Here's how the part is built. I have some questions about the finished solid (model axes, mm). A direction names the side the tool comes from. Coordinates: 2 decimals unless noted, no trailing zeros. Write each loop counter-clockwise with the first axis right and the second up, starting at its lowest first coordinate (ties: lowest second). Pieces come first, ordered by that corner, then holes. Notation, with made-up numbers: M 75.5,23.5 L 121.5,23.5 A14 ccw 121.5,37.5 Z; hole C 43.25,4.5 d11. An arc over 180 degrees is marked long. Use a Markdown table: item, result.
Solid Edge part; units mm, degrees
sketch "Sketch1" plane through (0, 0, 0) normal (0, -1, 0) x (1, 0, 0)
  line L0 (-16, -36) -> (16, -36)
  line L1 (16, -36) -> (16, 36)
  line L2 (16, 36) -> (-16, 36)
  line L3 (-16, 36) -> (-16, -36)
  line L4 (-20, -40) -> (20, -40)
  line L5 (20, -40) -> (20, 40)
  line L6 (20, 40) -> (-20, 40)
  line L7 (-20, 40) -> (-20, -40)
  dimension "D1" = 20
  dimension "D2" = 20
extrude "Protrusion1" add sketch "Sketch1" along normal mid plane 700
sketch "Sketch2" plane through (-20, 0, 0) normal (-1, 0, 0) x (0, -1, 0)
  line L0 (196, -40) -> (216, -40)
  line L1 (216, -40) -> (216, -35)
  line L2 (216, -35) -> (196, -35)
  line L3 (196, -35) -> (196, -40)
  line L4 (-284, -40) -> (-264, -40)
  line L5 (-264, -40) -> (-264, -35)
  line L6 (-264, -35) -> (-284, -35)
  line L7 (-284, -35) -> (-284, -40)
  dimension "D1" = 264
  dimension "D2" = 264
  dimension "D3" = 216
  dimension "D4" = 196
extrude "Cutout1" cut sketch "Sketch2" against normal through all
sketch "Sketch3" plane through (-20, 0, 0) normal (-1, 0, 0) x (0, -1, 0)
  circle A0 centre (-126, 10) radius 3.5
  circle A1 centre (34, 10) radius 3.5
  dimension "D1" = 126
  dimension "D2" = 126
extrude "Cutout2" cut sketch "Sketch3" against normal through all
sketch "Sketch4" plane through (-20, 0, 0) normal (-1, 0, 0) x (0, -1, 0)
  line L0 (350, 40) -> (313.5, 40)
  line L1 (313.5, 40) -> (313.5, 36)
  line L2 (313.5, 36) -> (346, 36)
  line L3 (346, 36) -> (346, 32)
  line L4 (346, 32) -> (350, 32)
  line L5 (350, 32) -> (350, 40)
  dimension "D1" = 350
  dimension "D2" = 313.5
  dimension "D3" = 346
  dimension "D4" = 346
extrude "Cutout3" cut sketch "Sketch4" against normal through all
mirror "Mirror1" about plane through (0, 0, 0) normal (0, 0, 1) of "Cutout3"
mirror "Mirror2" about plane through (0, 0, 0) normal (0, -1, 0) of "Cutout3", "Mirror1"
sketch "Sketch5" plane through (-20, 0, 0) normal (-1, 0, 0) x (0, 1, 0)
  circle A0 centre (-330, 0) radius 3
  circle A1 centre (-300, -25) radius 3
  circle A2 centre (-300, 25) radius 3
  dimension "D1" = 330
extrude "Cutout4" cut sketch "Sketch5" against normal through all
mirror "Mirror3" about plane through (0, 0, 0) normal (0, -1, 0) of "Cutout4"
sketch "Sketch6" plane through (-20, 0, 0) normal (-1, 0, 0) x (0, -1, 0)
  circle A0 centre (241, -27.5) radius 4
  circle A1 centre (241, -9.5) radius 3.25
  circle A2 centre (215, -27.5) radius 3.25
  circle A3 centre (215, -9.5) radius 4
  circle A4 centre (129, -9.5) radius 4
  circle A5 centre (103, -9.5) radius 3.25
  circle A6 centre (103, -27.5) radius 4
  circle A7 centre (129, -27.5) radius 3.25
extrude "Cutout5" cut sketch "Sketch6" against normal through all
sketch "Sketch7" plane through (-20, 0, 0) normal (-1, 0, 0) x (0, 1, 0)
  circle A0 centre (-172, 9.5) radius 8
extrude "Cutout6" cut sketch "Sketch7" against normal through all
properties material "AlSi7Mg"
1. Suppose I cut it at B-B on y = -56. Write out the boundary of the cut face in (x, z).
Answers follow:
| item | result |
|---|---|
| outline | M -20,-40 L 20,-40 L 20,40 L -20,40 Z; hole M -16,-36 L 16,-36 L 16,36 L -16,36 Z |
2. Will these pins go through, and if not, where does the flat tip stop? pin 1 Ø1.2 at (x, z) = (-4, 38.5) entering from +Y; pin 2 Ø2 at (x, y) = (18, -347.5) entering from +Z; pin 3 Ø3 at (x, y) = (18.5, 328) entering from -Z.
Answers follow:
| item | result |
|---|---|
| pin 1 | stops at y = 313.5 |
| pin 2 | stops at z = 32 |
| pin 3 | stops at z = -36 |
3. Suppose I cut it at A-A on x = -4. Write out the boundary of the cut face in (y, z), and give its area (3 significant figures).
Answers follow:
| item | result |
|---|---|
| outline | M -313.5,-40 L -216,-40 L -216,-36 L -313.5,-36 Z; M -313.5,36 L 313.5,36 L 313.5,40 L -313.5,40 Z; M -196,-40 L 264,-40 L 264,-36 L -196,-36 Z; M 284,-40 L 313.5,-40 L 313.5,-36 L 284,-36 Z |
| area | 4,860 mm2 |
4. Which directions (+Z, -Z, +X, -X, +Y, -Y) give clear straight access to the entire face, cutting with the end or side of a thin tool? Please do faces 1 (the face through (0, -264, -36)), 2 (the face through (0, -264, -40)).
Answers follow:
| item | result |
|---|---|
| face 1 | +Y, -Y |
| face 2 | -Z, +X, -X, +Y, -Y |
5. I need wall thicknesses on probe 1 along Y at (x, z) = (17, -9); probe 2 along Z at (x, y) = (-17.9, 300); probe 3 along X at (y, z) = (290, 2). Which ranges of each line are inside material? Lowest first, please.
Answers follow:
| item | result |
|---|---|
| probe 1 | y = -350 to -244.21, -237.79 to -218.97, -211.03 to -179.98, -164.02 to -132.97, -125.03 to -106.21, -99.79 to 350 |
| probe 2 | z = -40 to -28, -22 to 22, 28 to 40 |
| probe 3 | x = -20 to -16, 16 to 20 |
6. We'd pull the mould along Y, two halves only. Please class faces 3 (the face through (17.972, -179.992, -9.852)), 4 (the face through (0, 37, -36)): +Y half, -Y half, draft (parallel to the pull), parting line (faces both ways), or undercut.
Answers follow:
| item | result |
|---|---|
| face 3 | undercut |
| face 4 | draft |
